Design review of the part built by this model. Coordinates are the model's own, in mm. A direction names the side the tool comes from. Give positions to 0.01 mm unless a question says otherwise; leave off trailing zeros. Loops run counter-clockwise (first coordinate to the right, second up) from the corner with the lowest first, then second, coordinate; pieces in that order, holes last. Notation, with made-up numbers: (19.5, 9.5) -> (47.5, 9.5) arc R31 cw to (47.5, 45.5) -> close; hole circle Ø1 at (67.25, 83.5). An arc over 180 degrees is marked (long way). Use a Markdown table: item, result. Add a question column.
1. Add section B-B (x = 0). State the section outline as (y, z) points (3 decimals).
2. Add section A-A (z = 0). State the section outline as (x, y) points, and give its area (3 significant figures).
3. Add section D-D (z = -28.5). State the section outline as (x, y) points, and give its area (3 significant figures).
4. For pin 1 Ø3.5 at (y, z) = (-3.5, -75) entering from +X; pin 2 Ø1.1 at (y, z) = (-2, -74.5) entering from -X; pin 3 Ø1.1 at (y, z) = (-4, -72.5) entering from +X, all flat-tipped, find the tip position at first contact; note any pin that passes through.
5. To check wall thickness, follow line 1 (Z direction, x = -15.5, y = -4.65) (3 decimals); line 2 (Z direction, x = 18.5, y = -5.3) (3 decimals); line 3 (Z direction, x = 8.5, y = -4.65) (3 decimals). State the ranges of each line that lie inside material, in increasing order.
6. For faces 4 (the flat face through (-22, -3, -13)), 5 (the flat face through (15, -3, -69.799)), 6 (the flat face through (19.05, -3, 22)), 7 (the flat face through (-20, -3, -73.304)), list the 3-axis set-ups (+Z, -Z, +X, -X, +Y, -Y) from which the entire face can be reached by the end or side of a thin tool; tool diameter is ignored.
7. Draft analysis for pull direction X (two halves, no side actions). For faces 1 (the flat face through (0, 0, -46)), 2 (the flat face through (27.842, -3, -84)), 3 (the flat face through (-15.847, -3, -74)), state which applies: pulls with the +X half, pulls with the -X half, needs draft (parallel to the pull), parting line crosses it, or undercut.
8. Add section C-C (x = 20.5). State the section outline as (y, z) points.
```python
from build123d import *

# Parameters (mm, degrees)
F0_R     = 1.5
F0_R_2   = 7.5
F0_R_3   = 2
F0_W     = 12.7
F0_H     = 5.842
F0_R_4   = 7.7
F1_DEPTH = 5.842
F2_R     = 3.175
F4_DEPTH = 5.843
F5_R     = 2.0828
F6_DEPTH = 25.4


with BuildPart() as f1:
    # F0 (on Front) → F1 (new body)
    with BuildSketch(Plane.XZ):
        Polygon((22, 28.575), (-22, 28.575), (-22, -52.5018), (-27.842, -52.5018), (-27.842, -65.2018), (-22, -65.2018), (-22, -77.9018), (-27.842, -77.9018), (-27.842, -90.6018), (-22, -90.6018), (-22, -95.25), (22, -95.25), (22, -90.6018), (27.842, -90.6018), (27.842, -77.9018), (22, -77.9018), (22, -65.2018), (27.842, -65.2018), (27.842, -52.5018), (22, -52.5018), align=None)
        with Locations((-15.5, -87.0518)):
            Circle(F0_R, mode=Mode.SUBTRACT)
        with Locations((-15.5, -56.0518)):
            Circle(F0_R, mode=Mode.SUBTRACT)
        with Locations((0, -71.5518)):
            Circle(F0_R_2, mode=Mode.SUBTRACT)
        with Locations((15.5, -87.0518)):
            Circle(F0_R, mode=Mode.SUBTRACT)
        with Locations((15.5, -56.0518)):
            Circle(F0_R, mode=Mode.SUBTRACT)
        with Locations((-12.255778, -33.3375)):
            Circle(F0_R_3, mode=Mode.SUBTRACT)
        with Locations((-12.7, 22.225)):
            Rectangle(F0_W, F0_H, mode=Mode.SUBTRACT)
        with Locations((12.255778, -33.3375)):
            Circle(F0_R_3, mode=Mode.SUBTRACT)
        Circle(F0_R_4, mode=Mode.SUBTRACT)
        with Locations((12.7, 22.225)):
            Rectangle(F0_W, F0_H, mode=Mode.SUBTRACT)
    extrude(amount=F1_DEPTH)

    # F2
    f2_edges = [f1.edges().sort_by_distance(p)[0] for p in [
        (-22, -2.921, 28.575),
        (22, -2.921, 28.575),
    ]]
    fillet(f2_edges, radius=F2_R)

    # F3 (on face) → F4 (cut, through all)
    with BuildSketch(Plane.XZ.offset(5.842)):
        Polygon((-18.825, -69.7992), (-22, -69.7992), (-22, -73.3044), (-18.825, -73.3044), (-18.825, -75.52055), (-15.846875, -75.52055), (-15.846875, -73.3044), (-13.3545, -73.3044), (-13.3545, -69.7992), (-15.846875, -69.7992), (-15.846875, -67.58305), (-18.825, -67.58305), align=None)
        Polygon((22, -73.3044), (22, -69.7992), (18.825, -69.7992), (18.825, -67.58305), (15.846875, -67.58305), (15.846875, -69.7992), (13.3545, -69.7992), (13.3545, -73.3044), (15.846875, -73.3044), (15.846875, -75.52055), (18.825, -75.52055), (18.825, -73.3044), align=None)
    extrude(amount=-F4_DEPTH, mode=Mode.SUBTRACT)

    # F5 (on face) → F6 (cut)
    with BuildSketch(Plane.XZ.offset(5.842)):
        with Locations((0, 22.225)):
            Circle(F5_R)
    extrude(amount=-F6_DEPTH, mode=Mode.SUBTRACT)


solid = f1.part
```
Taken from the geometry:
| question | item | result |
|---|---|---|
| 1 | outline | (-5.842, -95.25) -> (0, -95.25) -> (0, -79.052) -> (-5.842, -79.052) -> close; (-5.842, -64.052) -> (0, -64.052) -> (0, -7.7) -> (-5.842, -7.7) -> close; (-5.842, 7.7) -> (0, 7.7) -> (0, 20.142) -> (-5.842, 20.142) -> close; (-5.842, 24.308) -> (0, 24.308) -> (0, 28.575) -> (-5.842, 28.575) -> close |
| 2 | outline | (-22, -5.84) -> (-7.7, -5.84) -> (-7.7, 0) -> (-22, 0) -> close; (7.7, -5.84) -> (22, -5.84) -> (22, 0) -> (7.7, 0) -> close |
| 2 | area | 167 mm^2 |
| 3 | outline | (-22, -5.84) -> (22, -5.84) -> (22, 0) -> (-22, 0) -> close |
| 3 | area | 257 mm^2 |
| 4 | pin 1 | stops at x = 22 |
| 4 | pin 2 | stops at x = -22 |
| 4 | pin 3 | stops at x = 13.35 |
| 5 | line 1 | z = -95.25 to -88.552, -85.552 to -73.304, -69.799 to -57.552, -54.552 to 19.304, 25.146 to 28.575 |
| 5 | line 2 | z = -95.25 to -75.521, -67.583 to 19.304, 25.146 to 28.575 |
| 5 | line 3 | z = -95.25 to 19.304, 25.146 to 28.575 |
| 6 | face 4 | +Z, -X, +Y, -Y |
| 6 | face 5 | +X, +Y, -Y |
| 6 | face 6 | +Y, -Y |
| 6 | face 7 | -X, +Y, -Y |
| 7 | face 1 | needs draft |
| 7 | face 2 | pulls with the +X half |
| 7 | face 3 | undercut |
| 8 | outline | (-5.84, -95.25) -> (0, -95.25) -> (0, -73.3) -> (-5.84, -73.3) -> close; (-5.84, -69.8) -> (0, -69.8) -> (0, 28.1) -> (-5.84, 28.1) -> close |
